Source: CAD feature listing. Evaluate the final solid. Frame: model axes, mm. A direction names the side the tool comes from. Give positions to 0.01 mm unless a question says otherwise; leave off trailing zeros. Order: outer loops, then holes, each group sorted by start corner. A loop starts at its lowest first (then second) coordinate and runs counter-clockwise, first axis right, second up. Notation, with made-up numbers: M 17.25,-7.5 L 29.25,-7.5 A25 cw 29.25,25.5 Z; hole C 29.25,-17 d11. An arc over 180 degrees is marked long. Answer in a Markdown table with one row per item. Add a question column.
(1) Material intervals for line 1 along Z through (x, y) = (10.5, -2); line 2 along Z through (x, y) = (18, -1.75); line 3 along X through (y, z) = (0.25, 14), sorted ascending.
(2) Pin query (flat end, axial travel): P1, Ø4, axis at x = 9, y = 1.5, coming from the +Z side; P2, Ø4, axis at x = 9, y = -1.5, coming from the -Z side; P3, Ø1.5, axis at y = 3.5, z = -5, coming from the -X side. Return the tip coordinate at first contact, or that it passes through.
(3) Section query A-A, the plane z = 43. Return loops of the section in (x, y), plus the area to 3 significant figures.
(4) Set-up query: faces 1 (the face through (14.556, -3.085, -59.082)), 2 (the face through (15, 0, -57.8)). Return all of +Z, -Z, +X, -X, +Y, -Y with unobstructed straight access to the full face (end or side cutting, diameter ignored); none if empty.
(5) Mould query, pull axis Z, two halves, no side actions, for faces 3 (the face through (9.39, -3.12, 58.58)), 4 (the face through (6.91, 0.03, 0.8)), 5 (the face through (15, 0, 57.8)), 6 (the face through (10.2, 0, 1)). Classes: pulls with the +Z half, pulls with the -Z half, needs draft (parallel to the pull), parting line crosses it, or undercut.
(6) Section query B-B, the plane y = -3.25. Return loops of the section in (x, z).
from build123d import *

# Parameters (mm, degrees)
FILLET003_R = 2.6


with BuildPart() as railfillet:
    # Sweep: sweep along a path in Sketch005
    with BuildLine(Plane.XZ) as sweep_path:
        Line((6.5, 0), (6.5, 57.5))
        ThreePointArc((6.5, 57.5), (7.671565, 60.328443), (10.500001, 61.500024))
        Line((10.500001, 61.500024), (18.500001, 61.500024))
    # Sketch011 → Sweep (sweep)
    with BuildSketch(Plane.XY):
        Polygon((10.2, 4.366273), (5.833727, 0), (10.2, -4.366273), align=None)
    sweep(path=sweep_path.line)

    # Fillet003
    fillet003_edges = [railfillet.edges().sort_by_distance(p)[0] for p in [
        (14.500005, 1.3e-05, 62.166285),
    ]]
    fillet(fillet003_edges, radius=FILLET003_R)


with BuildPart() as guide:
    # Part__Mirroring: instance of RailFillet
    add(railfillet.part.mirror(Plane(origin=(0, 0, 0), x_dir=(0, 1, 0), z_dir=(0, 0, 1))))

    # Fusion: union RailFillet
    add(railfillet.part)


solid = guide.part
Values follow:
| question | item | result |
|---|---|---|
| 1 | line 1 | z = -60.17 to -57.8, 57.8 to 60.17 |
| 1 | line 2 | z = -60.41 to -57.8, 57.8 to 60.41 |
| 1 | line 3 | x = 6.92 to 10.2 |
| 2 | P1 | stops at z = 61.09 |
| 2 | P2 | stops at z = -61.09 |
| 2 | P3 | stops at x = 8.58 |
| 3 | outline | M 7.67,-1.84 L 10.2,-4.37 L 10.2,4.37 L 7.67,1.84 A2.6 ccw Z |
| 3 | area | 17.6 mm² |
| 4 | face 1 | -Z, +X, -X, -Y |
| 4 | face 2 | +X, +Y, -Y |
| 5 | face 3 | pulls with the +Z half |
| 5 | face 4 | needs draft |
| 5 | face 5 | undercut |
| 5 | face 6 | undercut |
| 6 | outline | M 9.08,-57.5 A1.42 ccw 10.5,-58.92 L 18.5,-58.92 L 18.5,-57.8 L 10.5,-57.8 A0.3 cw 10.2,-57.5 L 10.2,57.5 A0.3 cw 10.5,57.8 L 18.5,57.8 L 18.5,58.92 L 10.5,58.92 A1.42 ccw 9.08,57.5 Z |
